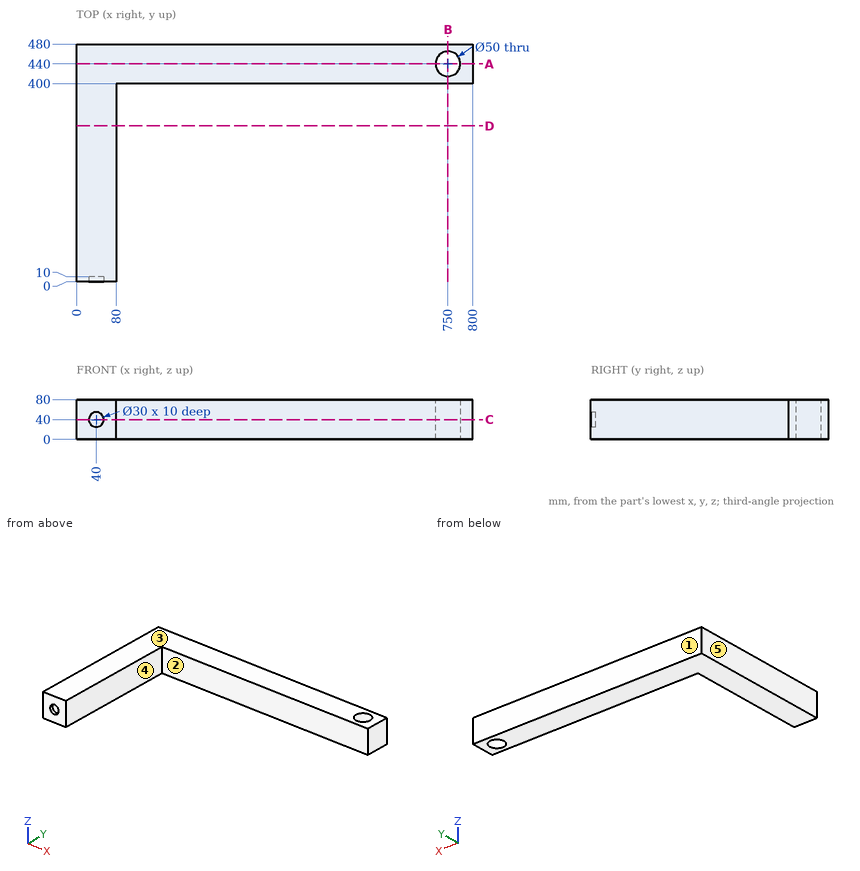
Answer from the drawing. Dimensions are ordinates in mm from the lowest x, y and z of the part. A direction names the side the tool comes from. Coordinates: 2 decimals unless noted, no trailing zeros. Loops run counter-clockwise (first coordinate to the right, second up) from the corner with the lowest first, then second, coordinate; pieces in that order, holes last. Notation, with made-up numbers: (17.25, -15) -> (40.25, -15) arc R24 cw to (40.25, 24) -> close; hole circle Ø8 at (43, -7). An arc over 180 degrees is marked (long way). Return JSON: item names as keys, results as strings.
Item 1: Find section C-C (z = 40). Determine the outline of the cut face in (x, y).
Answers:
{"outline": "(0, 0) -> (25, 0) -> (25, 10) -> (55, 10) -> (55, 0) -> (80, 0) -> (80, 400) -> (800, 400) -> (800, 480) -> (0, 480) -> close; hole circle Ø50 at (750, 440)"}
Item 2: Find section B-B (x = 750). Determine the outline of the cut face in (y, z), plus the area to 3 significant figures.
Answers:
{"outline": "(400, 0) -> (415, 0) -> (415, 80) -> (400, 80) -> close; (465, 0) -> (480, 0) -> (480, 80) -> (465, 80) -> close", "area": "2,400 mm2"}
Item 3: For a pull along X with two mould halves and no side action, classify the marked faces 3, 4 and 5 as +X half, -X half, draft (parallel to the pull), parting line (faces both ways), or undercut.
Answers:
{"face 3": "draft", "face 4": "+X half", "face 5": "-X half"}
Item 4: Flat-ended cylindrical pins translate along their axes: P1, Ø2, axis at y = 347, z = 28, coming from the +X side; P2, Ø24, axis at x = 269.5, z = 41, coming from the -Y side; P3, Ø24, axis at x = 40, z = 40, coming from the -Y side. Find the tip coordinate at first contact, or state that the pin passes through.
Answers:
{"P1": "stops at x = 80", "P2": "stops at y = 400", "P3": "stops at y = 10"}
Item 5: Find section A-A (y = 440). Determine the outline of the cut face in (x, z), plus the area to 3 significant figures.
Answers:
{"outline": "(0, 0) -> (725, 0) -> (725, 80) -> (0, 80) -> close; (775, 0) -> (800, 0) -> (800, 80) -> (775, 80) -> close", "area": "60,000 mm2"}
Item 6: For the marked faces 1 and 2, determine the directions among +Z, -Z, +X, -X, +Y, -Y from which every point of the face is accessible in a straight line to the end or side of a thin tool.
Answers:
{"face 1": "+Z, -Z, +X, -X, +Y", "face 2": "+Z, -Z, +X, -Y"}
Item 7: Find section D-D (y = 314.5). Determine the outline of the cut face in (x, z), plus the area to 3 significant figures.
Answers:
{"outline": "(0, 0) -> (80, 0) -> (80, 80) -> (0, 80) -> close", "area": "6,400 mm2"}
Item 8: Find the intervals of material crossed by probe 1 along Y at (x, z) = (750, 29.5); probe 2 along X at (y, z) = (2, 40); probe 3 along Y at (x, z) = (672, 48.5), in increasing order.
Answers:
{"probe 1": "y = 400 to 415, 465 to 480", "probe 2": "x = 0 to 25, 55 to 80", "probe 3": "y = 400 to 480"}
